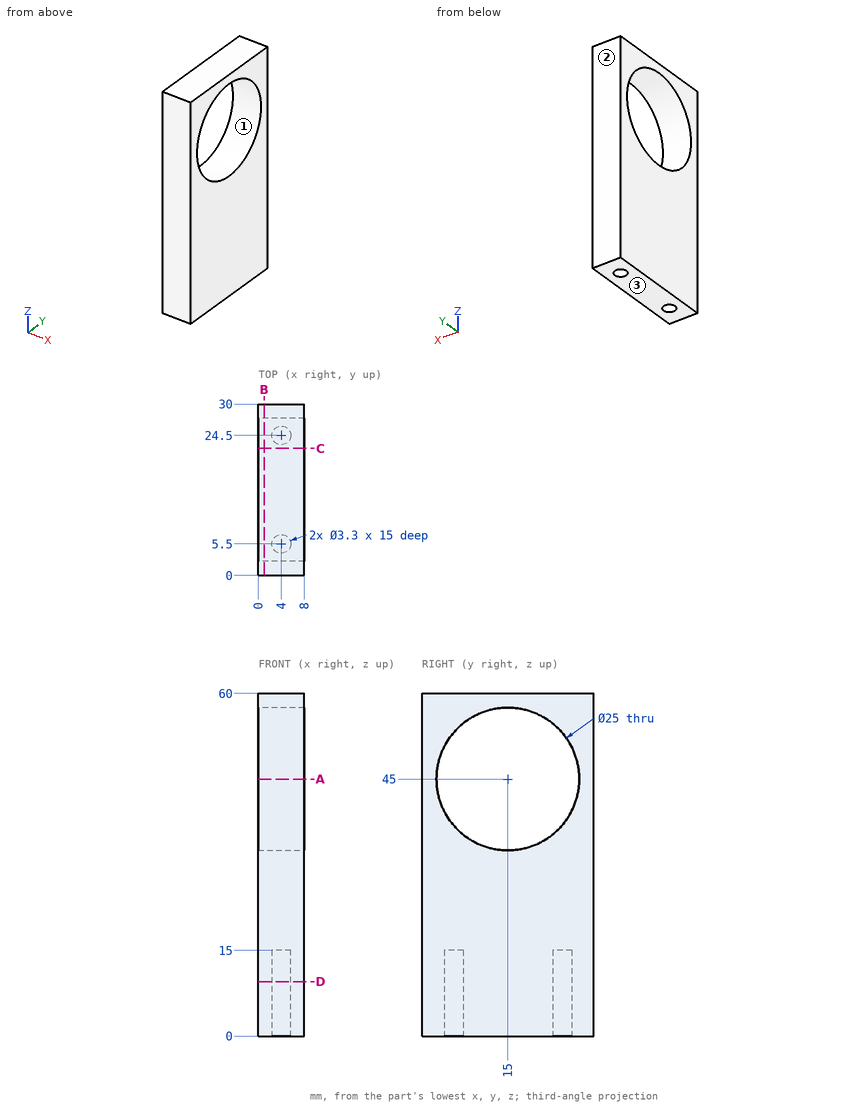
Here's the drawing with two shaded views (mm, measured from the low corner). I have some questions. Coordinates: 2 decimals unless noted, no trailing zeros. Loops run counter-clockwise (first coordinate to the right, second up) from the corner with the lowest first, then second, coordinate; pieces in that order, holes last. Notation, with made-up numbers: (37, 14) -> (44, 14) arc R5 cw to (44, 18) -> close; hole circle Ø2 at (-12, 64.5). An arc over 180 degrees is marked (long way). Answer as a JSON object with one key per item and string values.
1) If I drill on line 1 (Y direction, x = 4, z = 11.75); line 2 (Y direction, x = 5.75, z = 45); line 3 (X direction, y = 24.5, z = 6), over which ranges is the centre line in solid material (lowest first)?
Results:
{"line 1": "y = 0 to 3.85, 7.15 to 22.85, 26.15 to 30", "line 2": "y = 0 to 2.5, 27.5 to 30", "line 3": "x = 0 to 2.35, 5.65 to 8"}
2) Imagine slicing it at C-C (y = 22.25). Please give me the cut outline in (x, z).
Results:
{"outline": "(0, 0) -> (8, 0) -> (8, 34.82) -> (0, 34.82) -> close; (0, 55.18) -> (8, 55.18) -> (8, 60) -> (0, 60) -> close"}
3) For P1, Ø3.5, axis at x = 4, y = 24, coming from the -Z side; P2, Ø1, axis at x = 4.5, y = 5, coming from the -Z side, each with a flat end and sliding along its axis, tell me the tip position at first contact or that it passes through.
Results:
{"P1": "stops at z = 0", "P2": "stops at z = 15"}
4) Imagine slicing it at B-B (x = 1). Please give me the cut outline in (y, z).
Results:
{"outline": "(0, 0) -> (30, 0) -> (30, 60) -> (0, 60) -> close; hole circle Ø25 at (15, 45)"}
5) Imagine slicing it at A-A (z = 45). Please give me the cut outline in (x, y), then the cut area to 3 significant figures.
Results:
{"outline": "(0, 0) -> (8, 0) -> (8, 2.5) -> (0, 2.5) -> close; (0, 27.5) -> (8, 27.5) -> (8, 30) -> (0, 30) -> close", "area": "40.0 mm^2"}
6) Imagine slicing it at D-D (z = 9.5). Please give me the cut outline in (x, y).
Results:
{"outline": "(0, 0) -> (8, 0) -> (8, 30) -> (0, 30) -> close; hole circle Ø3.3 at (4, 5.5); hole circle Ø3.3 at (4, 24.5)"}
7) Thinking about a two-plate mould opening in Z: for the marked faces 1, 2 and 3, which applies, pulls with the +Z half, pulls with the -Z half, needs draft (parallel to the pull), parting line crosses it, or undercut?
Results:
{"face 1": "undercut", "face 2": "needs draft", "face 3": "pulls with the -Z half"}
